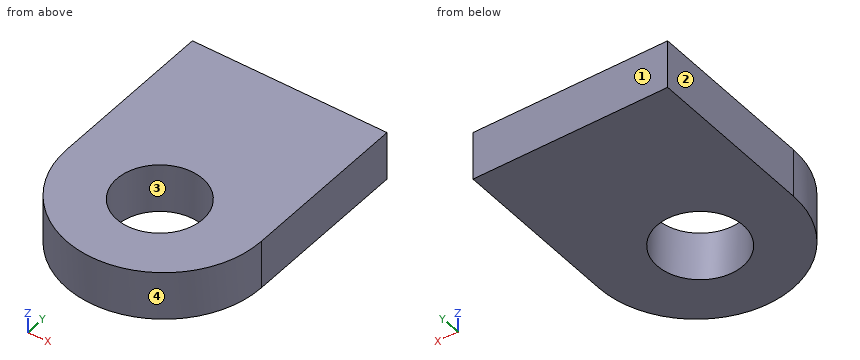
```python
from build123d import *

# Parameters (mm, degrees)
F0_W     = 50.8
F0_H     = 44.45
F1_DEPTH = 12.7
F2_R     = 11.241868
F3_DEPTH = 12.7


with BuildPart() as f1:
    # F0 (on Top) → F1 (new body)
    with BuildSketch(Plane.XY):
        with BuildLine():
            ThreePointArc((-25.4, -22.225), (0, -47.625), (25.4, -22.225))
            Line((25.4, -22.225), (-25.4, -22.225))
        make_face()
        Rectangle(F0_W, F0_H)
    extrude(amount=F1_DEPTH)

    # F2 (on Top) → F3 (cut)
    with BuildSketch(Plane.XY):
        with Locations((0, -23.683132)):
            Circle(F2_R)
    extrude(amount=F3_DEPTH, mode=Mode.SUBTRACT)


solid = f1.part
```
The model under review builds one solid part; all positions refer to its coordinate system, in mm. Face numbers are marked on the shaded views. Round coordinates to 2 decimals unless told otherwise and drop trailing zeros. Loops run counter-clockwise (first coordinate to the right, second up) from the corner with the lowest first, then second, coordinate; pieces in that order, holes last.
1) Consider section B-B on y = -20.5. State the section outline as (x, z) points.
Values follow:
outline: (-25.4, 0) - (-10.78, 0) - (-10.78, 12.7) - (-25.4, 12.7) - close; (10.78, 0) - (25.4, 0) - (25.4, 12.7) - (10.78, 12.7) - close
2) Wall thickness on line 1 along Y through (x, z) = (0, 4) (3 decimals); line 2 along Y through (x, z) = (-0.5, 3) (3 decimals); line 3 along X through (y, z) = (-29, 1.25): over which ranges is each line inside the solid? List them lowest first.
Values follow:
line 1: y = -47.625 to -34.925, -12.441 to 22.225
line 2: y = -47.62 to -34.914, -12.452 to 22.225
line 3: x = -24.48 to -9.91, 9.91 to 24.48
3) The part is to be moulded in two halves that separate along X. For the marked faces 1, 2, 3 and 4, say which applies: pulls with the +X half, pulls with the -X half, needs draft (parallel to the pull), parting line crosses it, or undercut.
Values follow:
face 1: needs draft
face 2: pulls with the -X half
face 3: undercut
face 4: parting line crosses it
4) Consider section C-C on z = 1.25. State the section outline as (x, y) points (3 decimals), then the cut area to 3 significant figures.
Values follow:
outline: (-25.4, -22.225) arc R25.4 ccw to (25.4, -22.225) - (25.4, 22.225) - (-25.4, 22.225) - close; hole circle Ø22.484 at (0, -23.683)
area: 2,870 mm2
5) Consider section D-D on x = -20. State the section outline as (y, z) points (3 decimals).
Values follow:
outline: (-37.883, 0) - (22.225, 0) - (22.225, 12.7) - (-37.883, 12.7) - close
6) Clearance check with flat-ended pins moving along their axes: P1, Ø6, axis at y = -30, z = 6.5, coming from the -X side; P2, Ø5, axis at x = -17.5, z = 4.5, coming from the -Y side. State where each tip first meets the part, or that it passes through.
Values follow:
P1: stops at x = -24.95
P2: stops at y = -42.72
7) Consider section A-A on x = 0. State the section outline as (y, z) points (3 decimals), then the cut area to 3 significant figures.
Values follow:
outline: (-47.625, 0) - (-34.925, 0) - (-34.925, 12.7) - (-47.625, 12.7) - close; (-12.441, 0) - (22.225, 0) - (22.225, 12.7) - (-12.441, 12.7) - close
area: 602 mm2
